Check sheet for the drawn part. Datum: minimum x, y, z corner. Units: mm. Round coordinates to 2 decimals unless told otherwise and drop trailing zeros. Write each loop counter-clockwise with the first axis right and the second up, starting at its lowest first coordinate (ties: lowest second). Pieces come first, ordered by that corner, then holes. Notation, with made-up numbers: (-6.5, 4) - (21.5, 4) arc R25 cw to (21.5, 33) - close; hole circle Ø1 at (-14, 18). An arc over 180 degrees is marked (long way). Answer as a JSON object with one key per item and string values.
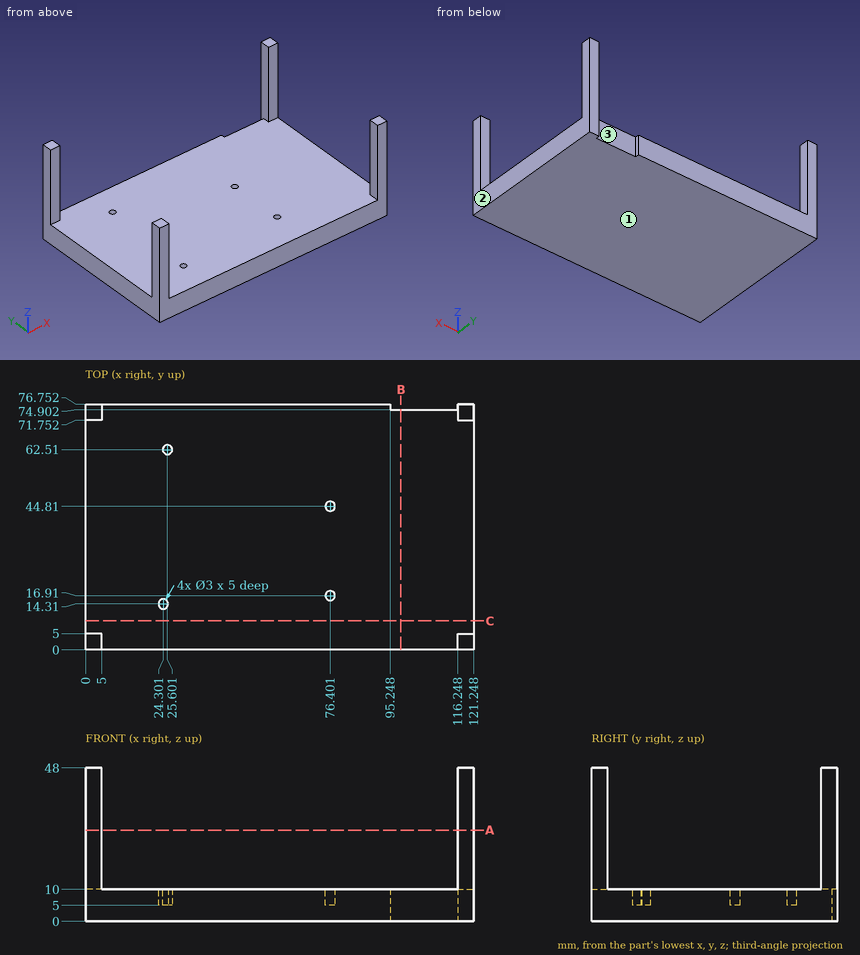
1. Cross-section at B-B (x = 98.5). Record the boundary of the cut face in (y, z).
Completed:
{"outline": "(0, 0) - (74.9, 0) - (74.9, 10) - (0, 10) - close"}
2. Mould release check, pull along X, two halves, no side actions. Record for the marked faces 1, 2 and 3: released by +X, released by -X, zero draft, split by the parting line, or undercut.
Completed:
{"face 1": "zero draft", "face 2": "released by +X", "face 3": "undercut"}
3. Go/stop test with flat-tipped pins: pin 1 (2.5 mm diameter, centred on x = 24.3, y = 14.31, fed in from +Z); pin 2 (8 mm diameter, centred on x = 102.5, z = 5, fed in from +Y); pin 3 (4 mm diameter, centred on x = 72, y = 38.5, fed in from +Z). Record where each tip stops, or that it passes through.
Completed:
{"pin 1": "stops at z = 5", "pin 2": "stops at y = 74.9", "pin 3": "stops at z = 10"}
4. Material ranges on probe 1 along X at (y, z) = (72, 45); probe 2 along Y at (x, z) = (25.5, 6) (1 decimal); probe 3 along Z at (x, y) = (71.5, 39), recorded low to high. Write a range as from..to.
Completed:
{"probe 1": "x = 0..5, 116.25..121.25", "probe 2": "y = 0..13.4, 15.2..61, 64..76.8", "probe 3": "z = 0..10"}
5. Cross-section at A-A (z = 28.5). Record the boundary of the cut face in (x, y), plus the area to 3 significant figures.
Completed:
{"outline": "(0, 0) - (5, 0) - (5, 5) - (0, 5) - close; (0, 71.75) - (5, 71.75) - (5, 76.75) - (0, 76.75) - close; (116.25, 0) - (121.25, 0) - (121.25, 5) - (116.25, 5) - close; (116.25, 71.75) - (121.25, 71.75) - (121.25, 76.75) - (116.25, 76.75) - close", "area": "100 mm^2"}
6. Cross-section at C-C (y = 9). Record the boundary of the cut face in (x, z).
Completed:
{"outline": "(0, 0) - (121.25, 0) - (121.25, 10) - (0, 10) - close"}
